Here's how the part is built. I have some questions about the finished solid (model axes, mm). Give positions to 0.01 mm unless a question says otherwise; leave off trailing zeros. Loops run counter-clockwise (first coordinate to the right, second up) from the corner with the lowest first, then second, coordinate; pieces in that order, holes last.
Q1. Suppose I cut it at C-C (y = 0). List the corners of the cut face in (x, z) for me (3 decimals).
Q2. I need wall thicknesses on probe 1 along Y at (x, z) = (-1.5, 0.2); probe 2 along X at (y, z) = (29.5, 0.9); probe 3 along X at (y, z) = (-31, 2.35). Which ranges of each line are inside material? Lowest first, please.
Q3. Suppose I cut it at A-A (x = 0). List the corners of the cut face in (y, z) for me (3 decimals), and give its area (3 significant figures).
Q4. Suppose I cut it at B-B (z = 0.9). List the corners of the cut face in (x, y) for me (3 decimals), and give its area (3 significant figures).
```python
from build123d import *

# Parameters (mm, degrees)
SKETCH1_R                                    = 2.5527
BOSS_EXTRUDE1_DEPTH                          = 3.175
CSK_FOR_1_4_FLAT_HEAD_SOCKET_CAP_SCR_2_COUNT = 2
CSK_FOR_1_4_FLAT_HEAD_SOCKET_CAP_SCR_2_PITCH = 25.4
CSK_FOR_1_4_FLAT_HEAD_SOCKET_CAP_SCR_3_COUNT = 2
CSK_FOR_1_4_FLAT_HEAD_SOCKET_CAP_SCR_3_PITCH = 50.8


with BuildPart() as part:
    # Sketch1 → Boss-Extrude1 (new body)
    with BuildSketch(Plane.XY):
        with BuildLine():
            Line((-22.225, 44.45), (22.225, 44.45))
            ThreePointArc((22.225, 44.45), (28.960192091, 41.660192091), (31.75, 34.925))
            Line((31.75, 34.925), (31.75, -34.925))
            ThreePointArc((31.75, -34.925), (28.960192091, -41.660192091), (22.225, -44.45))
            Line((22.225, -44.45), (-22.225, -44.45))
            ThreePointArc((-22.225, -44.45), (-28.960192091, -41.660192091), (-31.75, -34.925))
            Line((-31.75, -34.925), (-31.75, 34.925))
            ThreePointArc((-31.75, 34.925), (-28.960192091, 41.660192091), (-22.225, 44.45))
        make_face()
        with Locations((0, 25.4)):
            Circle(SKETCH1_R, mode=Mode.SUBTRACT)
        Circle(SKETCH1_R, mode=Mode.SUBTRACT)
        with Locations((0, -25.4)):
            Circle(SKETCH1_R, mode=Mode.SUBTRACT)
    extrude(amount=BOSS_EXTRUDE1_DEPTH)

    # Sketch2 → CSK for 1/4 Flat Head Socket Cap Screw1 (revolve, cut)
    with BuildSketch(Plane(origin=(0, 25.4, 3.175), x_dir=(0, -1, 0), z_dir=(1, 0, 0))):
        Polygon((0, 0), (0, 3.175), (3.3782, 3.175), (3.3782, 3.871564875), (6.7437, 0), align=None)
    csk_for_1_4_flat_head_socket_cap_screw1 = revolve(axis=Axis((0, 25.4, 9.525), (0, 0, -1)), mode=Mode.SUBTRACT)

    # CSK for 1_4 Flat Head Socket Cap Scr 2: CSK for 1/4 Flat Head Socket Cap Screw1 ×2
    with Locations(*[(0, -i * CSK_FOR_1_4_FLAT_HEAD_SOCKET_CAP_SCR_2_PITCH, 0) for i in range(1, CSK_FOR_1_4_FLAT_HEAD_SOCKET_CAP_SCR_2_COUNT)]):
        add(csk_for_1_4_flat_head_socket_cap_screw1, mode=Mode.SUBTRACT)

    # CSK for 1_4 Flat Head Socket Cap Scr 3: CSK for 1/4 Flat Head Socket Cap Screw1 ×2
    with Locations(*[(0, -i * CSK_FOR_1_4_FLAT_HEAD_SOCKET_CAP_SCR_3_PITCH, 0) for i in range(1, CSK_FOR_1_4_FLAT_HEAD_SOCKET_CAP_SCR_3_COUNT)]):
        add(csk_for_1_4_flat_head_socket_cap_screw1, mode=Mode.SUBTRACT)


solid = part.part
```
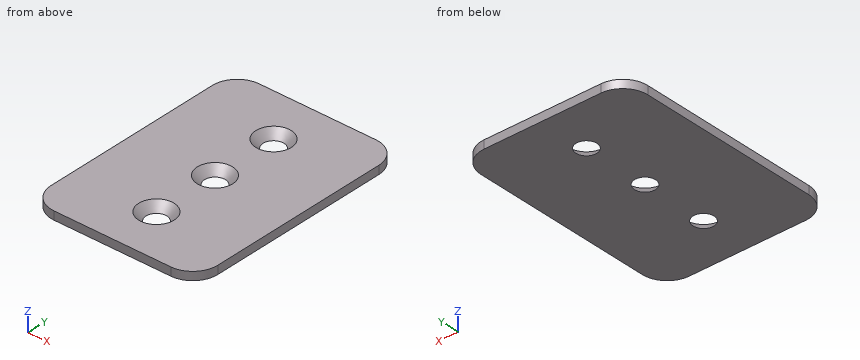
Solutions:
1. outline: (-31.75, 0) - (-3.984, 0) - (-6.744, 3.175) - (-31.75, 3.175) - close; (3.984, 0) - (31.75, 0) - (31.75, 3.175) - (6.744, 3.175) - close
2. probe 1: y = -44.45 to -29.28, -21.52 to -3.88, 3.88 to 21.52, 29.28 to 44.45
2. probe 2: x = -31.75 to -2.43, 2.43 to 31.75
2. probe 3: x = -31.75 to -2.23, 2.23 to 31.75
3. outline: (-44.45, 0) - (-29.384, 0) - (-32.144, 3.175) - (-44.45, 3.175) - close; (-21.416, 0) - (-3.984, 0) - (-6.744, 3.175) - (-18.656, 3.175) - close; (3.984, 0) - (21.416, 0) - (18.656, 3.175) - (6.744, 3.175) - close; (29.384, 0) - (44.45, 0) - (44.45, 3.175) - (32.144, 3.175) - close
3. area: 180 mm2
4. outline: (-31.75, -34.925) arc R9.525 ccw to (-22.225, -44.45) - (22.225, -44.45) arc R9.525 ccw to (31.75, -34.925) - (31.75, 34.925) arc R9.525 ccw to (22.225, 44.45) - (-22.225, 44.45) arc R9.525 ccw to (-31.75, 34.925) - close; hole circle Ø9.532 at (0, -25.4); hole circle Ø9.532 at (0, 0); hole circle Ø9.532 at (0, 25.4)
4. area: 5,350 mm2
